from build123d import *

# Parameters (mm, degrees)
F4_DEPTH = 3.5
F6_D     = 6
F6_DEPTH = 25
F6_TIP   = 1.8025818571


with BuildPart() as f1:
    # F0 (on Front) → F1 (revolve)
    with BuildSketch(Plane.XZ):
        Polygon((0, 10), (0, 0), (253.3, 0), (253.3, 9), (117.3, 9), (117.3, 9.5), (117.3, 11), (84.8, 11), (84.8, 12.5), (44.8, 12.5), (44.8, 11), (12.3, 11), (12.3, 10), (5.3, 10), (5.3, 9.5), (4, 9.5), (4, 10), align=None)
    revolve(axis=Axis((126.65, 0, 0), (1, 0, 0)))

    # F3 (on offset) → F4 (cut)
    with BuildSketch(Plane.XY.offset(9)):
        with BuildLine():
            Line((178.3, -3), (253.3, -3))
            Line((253.3, -3), (253.3, 3))
            Line((253.3, 3), (178.3, 3))
            ThreePointArc((178.3, 3), (175.3, 0), (178.3, -3))
        make_face()
    extrude(amount=-F4_DEPTH, mode=Mode.SUBTRACT)

    # F6
    with Locations(Plane.YZ.offset(253.3)):
        with Locations((0, 0)):
            Hole(F6_D / 2, depth=F6_DEPTH)
            with Locations((0, 0, -(F6_DEPTH + F6_TIP / 2))):  # 118° drill point
                Cone(0, F6_D / 2, F6_TIP, mode=Mode.SUBTRACT)


solid = f1.part
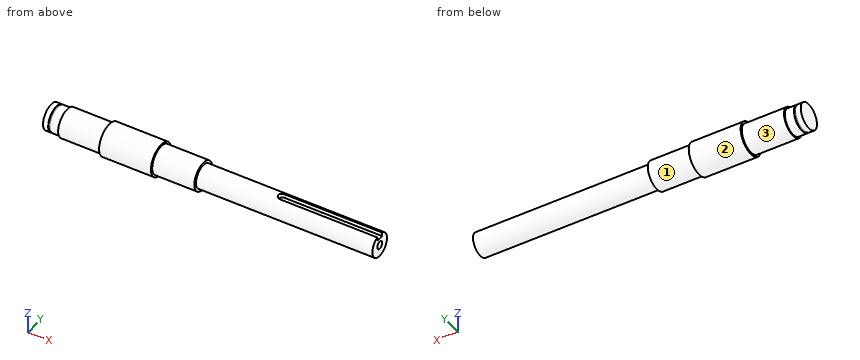
Geometry: final body of the model. Coordinates: model frame, mm. Face numbers are marked on the shaded views. A direction names the side the tool comes from. Round coordinates to 2 decimals unless told otherwise and drop trailing zeros. Loops run counter-clockwise (first coordinate to the right, second up) from the corner with the lowest first, then second, coordinate; pieces in that order, holes last.
Q1. Section B-B on y = 6.75. Return loops of the section in (x, z), plus the area to 3 significant figures.
Q2. Section D-D on y = -6. Return loops of the section in (x, z), plus the area to 3 significant figures.
Q3. Section A-A on x = 126.5. Return loops of the section in (y, z).
Q4. Access query for the marked faces 1, 2 and 3. Directions: +Z, -Z, +X, -X, +Y, -Y. A direction counts if a zero-diameter tool reaches every point of the face in a straight line with its end or side. Return the directions, or none.
Q5. Pin query (flat end, axial travel): P1, Ø8, axis at x = 217.5, z = -8, coming from the -Y side; P2, Ø3, axis at y = 7.5, z = 8.5, coming from the +X side; P3, Ø10, axis at x = 147, z = 8.5, coming from the +Y side. Return the tip coordinate at first contact, or that it passes through.
Q6. Material intervals for L1, parallel to Y at x = 238.5, z = 0; L2, parallel to Z at x = 245.5, y = 0; L3, parallel to X at y = -0.75, z = 9.5, sorted ascending.
Q7. Section C-C on x = 186. Return loops of the section in (y, z), plus the area to 3 significant figures.
Evaluation:
1. outline: (0, -7.38) - (4, -7.38) - (4, -6.68) - (5.3, -6.68) - (5.3, -7.38) - (12.3, -7.38) - (12.3, -8.69) - (44.8, -8.69) - (44.8, -10.52) - (84.8, -10.52) - (84.8, -8.69) - (117.3, -8.69) - (117.3, -5.95) - (253.3, -5.95) - (253.3, 5.95) - (117.3, 5.95) - (117.3, 8.69) - (84.8, 8.69) - (84.8, 10.52) - (44.8, 10.52) - (44.8, 8.69) - (12.3, 8.69) - (12.3, 7.38) - (5.3, 7.38) - (5.3, 6.68) - (4, 6.68) - (4, 7.38) - (0, 7.38) - close
1. area: 3,770 mm2
2. outline: (0, -8) - (4, -8) - (4, -7.37) - (5.3, -7.37) - (5.3, -8) - (12.3, -8) - (12.3, -9.22) - (44.8, -9.22) - (44.8, -10.97) - (84.8, -10.97) - (84.8, -9.22) - (117.3, -9.22) - (117.3, -6.71) - (253.3, -6.71) - (253.3, 6.71) - (117.3, 6.71) - (117.3, 9.22) - (84.8, 9.22) - (84.8, 10.97) - (44.8, 10.97) - (44.8, 9.22) - (12.3, 9.22) - (12.3, 8) - (5.3, 8) - (5.3, 7.37) - (4, 7.37) - (4, 8) - (0, 8) - close
2. area: 4,100 mm2
3. outline: circle Ø18 at (0, 0)
4. face 1: +X
4. face 2: +X, -X
4. face 3: -X
5. P1: stops at y = -8.06
5. P2: stops at x = 117.3
5. P3: stops at y = 8.29
6. L1: y = -9 to -3, 3 to 9
6. L2: z = -9 to -3, 3 to 5.5
6. L3: x = 0 to 4, 5.3 to 117.3
7. outline: (-3, 5.5) - (-3, 8.49) arc R9 ccw (long way) to (3, 8.49) - (3, 5.5) - close
7. area: 234 mm2
